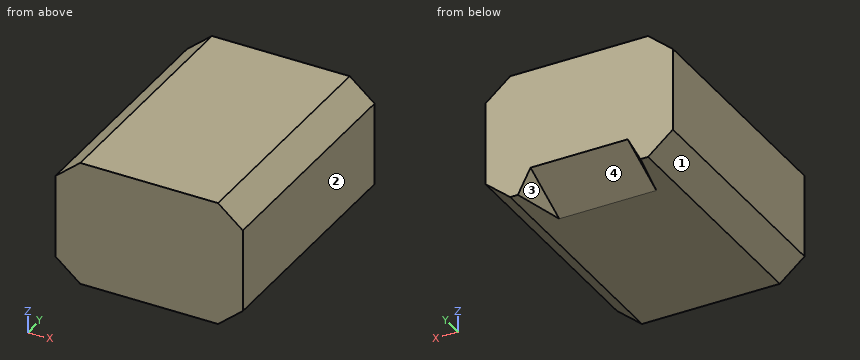
from build123d import *
from OCP.BRepFilletAPI import BRepFilletAPI_MakeChamfer

# Parameters (mm, degrees)
ESQUISSE1_W             = 270
ESQUISSE1_H             = 180
BOSS_EXTRU_1_DEPTH      = 345
CHANFREIN1_SIZE         = 30
CHANFREIN1_SIZE2        = 35.752607778
ENL_V_MAT_EXTRU_1_DEPTH = 90
CHANFREIN2_SIZE         = 20
CHANFREIN2_SIZE_2       = 34.641016151


with BuildPart() as part:
    # Esquisse1 → Boss.-Extru.1 (new body)
    with BuildSketch(Plane(origin=(0, 0, 0), x_dir=(1, 0, 0), z_dir=(0, 1, 0))):
        Rectangle(ESQUISSE1_W, ESQUISSE1_H)
    extrude(amount=BOSS_EXTRU_1_DEPTH)

    # Chanfrein1: one chamfer whose edges measure the first distance from different faces: ONE call of the kernel's chamfer builder (chamfer() names one face for all edges)
    chanfrein1_edges_1 = [part.edges().sort_by_distance(p)[0] for p in [
        (135, 172.5, 90),
        (135, 172.5, -90),
    ]]
    chanfrein1_side_1 = [part.faces().sort_by_distance(p)[0] for p in [
        (135, 172.5, 0),
    ]]
    chanfrein1_edges_2 = [part.edges().sort_by_distance(p)[0] for p in [
        (-135, 172.5, 90),
        (-135, 172.5, -90),
    ]]
    chanfrein1_side_2 = [part.faces().sort_by_distance(p)[0] for p in [
        (-135, 172.5, 0),
    ]]
    chanfrein1 = BRepFilletAPI_MakeChamfer(part.part.solid().wrapped)
    for e in chanfrein1_edges_1:
        chanfrein1.Add(CHANFREIN1_SIZE, CHANFREIN1_SIZE2, e.wrapped, chanfrein1_side_1[0].wrapped)  # the first distance lies on this face
    for e in chanfrein1_edges_2:
        chanfrein1.Add(CHANFREIN1_SIZE, CHANFREIN1_SIZE2, e.wrapped, chanfrein1_side_2[0].wrapped)  # the first distance lies on this face
    add(Compound.cast(chanfrein1.Shape()), mode=Mode.REPLACE)

    # Esquisse2 → Enlèv. mat.-Extru.1 (cut, symmetric)
    with BuildSketch(Plane(origin=(0, 0, 0), x_dir=(0, 0, -1), z_dir=(1, 0, 0))):
        Polygon((55, 345), (255, 345), (255, -83.901384102), align=None)
    extrude(amount=ENL_V_MAT_EXTRU_1_DEPTH, both=True, mode=Mode.SUBTRACT)

    # Chanfrein2
    # the kernel refuses this chamfer: 34.641016151, 20 mm, written as the material it adds along each edge
    with BuildSketch(Plane(origin=(90, 188.719606983, -127.874744083), x_dir=(-0.9983227437537926, -0.02446700349407226, 0.05246965831716883), z_dir=(0, 0.9063077870366479, 0.422618261740704))) as chanfrein2_piece_1_section:
        Polygon((CHANFREIN2_SIZE * 0.998322743754, -CHANFREIN2_SIZE * 0.0578938624027), (-CHANFREIN2_SIZE_2 * 0.0578938624033, -CHANFREIN2_SIZE_2 * 0.998322743765), (0, 0), align=None)
    chanfrein2_piece_1 = extrude(amount=262.055614234, mode=Mode.PRIVATE)
    chanfrein2_piece_1 = split(chanfrein2_piece_1, bisect_by=Plane(origin=(82.381838985, 345, -77.051948242), z_dir=(0, -1, 0)), keep=Keep.TOP, mode=Mode.PRIVATE)
    chanfrein2_piece_1 = split(chanfrein2_piece_1, bisect_by=Plane(origin=(82.381838985, 317.232813397, -90), z_dir=(0, 0, 1)), keep=Keep.TOP, mode=Mode.PRIVATE)
    add(chanfrein2_piece_1)
    with BuildSketch(Plane(origin=(-90, 188.719606983, -127.874744083), x_dir=(-0.0193267656127005, 0.42253932536473243, -0.906138507432097), z_dir=(0, 0.9063077870366479, 0.422618261740704))) as chanfrein2_piece_2_section:
        Polygon((CHANFREIN2_SIZE_2 * 0.999813220633, -CHANFREIN2_SIZE_2 * 0.0193267656129), (-CHANFREIN2_SIZE * 0.0193267656127, -CHANFREIN2_SIZE * 0.999813220622), (0, 0), align=None)
    chanfrein2_piece_2 = extrude(amount=262.055614234, mode=Mode.PRIVATE)
    chanfrein2_piece_2 = split(chanfrein2_piece_2, bisect_by=Plane(origin=(-82.381838985, 345, -77.051948242), z_dir=(0, -1, 0)), keep=Keep.TOP, mode=Mode.PRIVATE)
    chanfrein2_piece_2 = split(chanfrein2_piece_2, bisect_by=Plane(origin=(-82.381838985, 317.232813397, -90), z_dir=(0, 0, 1)), keep=Keep.TOP, mode=Mode.PRIVATE)
    add(chanfrein2_piece_2)


solid = part.part
Read the model definition and answer for the solid it produces. Units are mm, in the model's axes. Face numbers are marked on the shaded views. Give positions to 0.01 mm unless a question says otherwise; leave off trailing zeros. Write each loop counter-clockwise with the first axis right and the second up, starting at its lowest first coordinate (ties: lowest second). Pieces come first, ordered by that corner, then holes. Notation, with made-up numbers: (24.5, 11.25) - (81.5, 11.25) arc R25 ccw to (81.5, 29.25) - close; hole circle Ø9 at (71, 78.5). An arc over 180 degrees is marked (long way). Use CSV: the item, a comma, the result in double quotes. Start each with the question number.
Item 1: The part is cut by section D-D, the plane x = 112.5. Give the vertices of the cut face in (y, z).
Item 2: The mould has two halves that part along X. Classify the marked faces 1, 2, 3 and 4: pulls with the +X half, pulls with the -X half, needs draft (parallel to the pull), parting line crosses it, or undercut.
Item 3: The part is cut by section C-C, the plane x = -1. Give the vertices of the cut face in (y, z).
Item 4: The part is cut by section A-A, the plane y = 204. Give the vertices of the cut face in (x, z).
Item 5: Consider line 1 (X direction, y = 152, z = 78); line 2 (Z direction, x = -104.5, y = 80); line 3 (Z direction, x = 107, y = 260.5). Determine where each line is inside the solid, lowest interval first.
Item 6: Flat-ended cylindrical pins translate along their axes: P1, Ø12, axis at x = 100.5, z = -0.5, coming from the -Y side; P2, Ø1.5, axis at y = 182.5, z = -71.5, coming from the +X side. Find the tip coordinate at first contact, or state that the pin passes through.
Item 7: The part is cut by section B-B, the plane z = -77. Give the vertices of the cut face in (x, y).
Taken from the geometry:
1,outline,"(0, -78.88) - (345, -78.88) - (345, 78.88) - (0, 78.88) - close"
2,face 1,"pulls with the -X half"
2,face 2,"pulls with the +X half"
2,face 3,"undercut"
2,face 4,"undercut"
3,outline,"(0, -90) - (269.94, -90) - (345, -55) - (345, 90) - (0, 90) - close"
4,outline,"(-135, -60) - (-99.25, -90) - (99.25, -90) - (135, -60) - (135, 60) - (99.25, 90) - (-99.25, 90) - (-135, 60) - close"
5,line 1,"-113.55 to 113.55"
5,line 2,"-85.59 to 85.59"
5,line 3,"-83.49 to 83.49"
6,P1,"y = 0"
6,P2,"x = 122.19"
7,outline,"(-114.74, 0) - (114.74, 0) - (114.74, 345) - (81.51, 345) - (70, 297.82) - (-70, 297.82) - (-81.51, 345) - (-114.74, 345) - close"
